Verification items for the finished model (mm, model axes). A direction names the side the tool comes from. Give positions to 0.01 mm unless a question says otherwise; leave off trailing zeros. Write each loop counter-clockwise with the first axis right and the second up, starting at its lowest first coordinate (ties: lowest second). Pieces come first, ordered by that corner, then holes. Notation, with made-up numbers: (-38.5, -23) - (-25.5, -23) arc R21 ccw to (-25.5, -17) - close; hole circle Ø4 at (0, 37.5). An arc over 180 degrees is marked (long way). Answer as a JSON object with one key per item and string values. Group by question number.
Item 1: Sectioned sample at A-A, the plane y = -1.5. Record the boundary of the cut face in (x, z), and give its area (3 significant figures).
Item 2: Go/stop test with a flat-tipped pin: pin 1 (0.9 mm diameter, centred on x = 0, y = 2, fed in from -Z). Record where the tip stops, or that it passes through.
Item 3: Tool access check on faces 1 (the face through (0, 3, -0.953)), 2 (the face through (-0.83, 2.96, 0.47)), 3 (the face through (0.83, 2.96, -0.47)). Record the directions out of +Z, -Z, +X, -X, +Y, -Y that give a thin tool (end or side, any length) a straight path to the whole face; none if there is none.
Item 4: Sectioned sample at B-B, the plane z = -0.5. Record the boundary of the cut face in (x, y), and give its area (3 significant figures).
Item 5: Sectioned sample at D-D, the plane y = 4.5. Record the boundary of the cut face in (x, z), and give its area (3 significant figures).
Item 6: Scan lines: line 1 along Y through (x, z) = (-0.5, -3); line 2 along Z through (x, y) = (-3.25, -1); line 3 along Z through (x, y) = (3.5, -4.75). Record each from-to range of solid material in increasing order. Write a range as [from, to].
Item 7: Sectioned sample at C-C, the plane x = -1.25. Record the boundary of the cut face in (y, z), and give its area (3 significant figures).
```python
from build123d import *

# Parameters (mm, degrees)
BOSS_EXTRUDE1_DEPTH = 6
BOSS_EXTRUDE2_DEPTH = 8


with BuildPart() as part:
    # Sketch1 → Boss-Extrude1 (new body)
    with BuildSketch(Plane(origin=(0, 0, 0), x_dir=(1, 0, 0), z_dir=(0, 1, 0))):
        Polygon((1.1, 0), (0.55, 0.952627944), (-0.55, 0.952627944), (-1.1, 0), (-0.55, -0.952627944), (0.55, -0.952627944), align=None)
    extrude(amount=BOSS_EXTRUDE1_DEPTH)

    # Sketch2 → Boss-Extrude2 (add)
    with BuildSketch(Plane.XZ):
        Polygon((3.7, 0), (1.85, 3.204293994), (-1.85, 3.204293994), (-3.7, 0), (-1.85, -3.204293994), (1.85, -3.204293994), align=None)
    extrude(amount=BOSS_EXTRUDE2_DEPTH)


solid = part.part
```
Geometry check:
{
 "1": {"outline": "(-3.7, 0) - (-1.85, -3.2) - (1.85, -3.2) - (3.7, 0) - (1.85, 3.2) - (-1.85, 3.2) - close", "area": "35.6 mm^2"},
 "2": {"pin 1": "z = -0.95"},
 "3": {"face 1": "-Z, +X, -X, +Y", "face 2": "+Z, -X, +Y", "face 3": "-Z, +X, +Y"},
 "4": {"outline": "(-3.41, -8) - (3.41, -8) - (3.41, 0) - (0.81, 0) - (0.81, 6) - (-0.81, 6) - (-0.81, 0) - (-3.41, 0) - close", "area": "64.3 mm^2"},
 "5": {"outline": "(-1.1, 0) - (-0.55, -0.95) - (0.55, -0.95) - (1.1, 0) - (0.55, 0.95) - (-0.55, 0.95) - close", "area": "3.14 mm^2"},
 "6": {"line 1": "[-8, 0]", "line 2": "[-0.78, 0.78]", "line 3": "[-0.35, 0.35]"},
 "7": {"outline": "(-8, -3.2) - (0, -3.2) - (0, 3.2) - (-8, 3.2) - close", "area": "51.3 mm^2"}
}
